```python
from build123d import *

# Parameters (mm, degrees)
BOSS_EXTRUDE1_DEPTH       = 18
SKETCH2_W                 = 22.6
SKETCH2_H                 = 12.7
CUT_EXTRUDE1_DEPTH        = 10
F_4_CLEARANCE_HOLE3_D     = 3.2639
F_4_CLEARANCE_HOLE3_DEPTH = 1.59


with BuildPart() as part:
    # Sketch1 → Boss-Extrude1 (new body)
    with BuildSketch(Plane.XY):
        Polygon((10, -20), (0, -20), (0, 0), (40, 0), (40, -20), (30, -20), (30, -18.41), (38.41, -18.41), (38.41, -1.59), (1.59, -1.59), (1.59, -18.41), (10, -18.41), align=None)
    extrude(amount=BOSS_EXTRUDE1_DEPTH)

    # Sketch2 → Cut-Extrude1 (cut)
    with BuildSketch(Plane(origin=(0, 0, 0), x_dir=(1, 0, 0), z_dir=(0, 1, 0))):
        with Locations((20, -6.35)):
            Rectangle(SKETCH2_W, SKETCH2_H)
    extrude(amount=-CUT_EXTRUDE1_DEPTH, mode=Mode.SUBTRACT)

    # #4 Clearance Hole3
    with Locations(Plane(origin=(0, -18.41, 0), x_dir=(1, 0, 0), z_dir=(0, 1, 0))):
        with Locations((5.795, -9), (34.205, -9)):
            Hole(F_4_CLEARANCE_HOLE3_D / 2, depth=F_4_CLEARANCE_HOLE3_DEPTH)


solid = part.part
```
Geometry: final body of the model. Coordinates: model frame, mm. A direction names the side the tool comes from. Coordinates: 2 decimals unless noted, no trailing zeros. Order: outer loops, then holes, each group sorted by start corner. A loop starts at its lowest first (then second) coordinate and runs counter-clockwise, first axis right, second up. Notation, with made-up numbers: (40, 86) -> (54, 86) arc R20 cw to (54, 99) -> close; hole circle Ø10 at (-38, 58). An arc over 180 degrees is marked (long way). Answer in a Markdown table with one row per item.
Item 1: Access query for faces 1 (the flat face through (4, -18.41, 9)), 2 (the cylindrical face through (7.09, -19.22, 9.99)), 3 (the flat face through (8.7, -1, 6)), 4 (the flat face through (10, -19, 9)), 5 (the flat face through (4, -20, 9)). Directions: +Z, -Z, +X, -X, +Y, -Y. A direction counts if a zero-diameter tool reaches every point of the face in a straight line with its end or side. Return the directions, or none.
Return value:
| item | result |
|---|---|
| face 1 | +Z, -Z |
| face 2 | -Y |
| face 3 | -Z, +Y |
| face 4 | +Z, -Z, -Y |
| face 5 | +Z, -Z, +X, -X, -Y |
Item 2: Contact query for a flat-ended pin moving along its axis: P1, Ø0.8, axis at x = 24.5, y = -1, coming from the -Z side. Output: stop coordinate, or through.
Return value:
| item | result |
|---|---|
| P1 | stops at z = 12.7 |
Item 3: Section D-D on z = 9. Output: boundary loops of the cut face in (x, y), plus the area to 3 significant figures.
Return value:
| item | result |
|---|---|
| outline | (0, -20) -> (4.16, -20) -> (4.16, -18.41) -> (1.59, -18.41) -> (1.59, -1.59) -> (8.7, -1.59) -> (8.7, 0) -> (0, 0) -> close; (7.43, -20) -> (10, -20) -> (10, -18.41) -> (7.43, -18.41) -> close; (30, -20) -> (32.57, -20) -> (32.57, -18.41) -> (30, -18.41) -> close; (31.3, -1.59) -> (38.41, -1.59) -> (38.41, -18.41) -> (35.84, -18.41) -> (35.84, -20) -> (40, -20) -> (40, 0) -> (31.3, 0) -> close |
| area | 103 mm² |
Item 4: Section C-C on y = -9.5. Output: boundary loops of the cut face in (x, z), plus the area to 3 significant figures.
Return value:
| item | result |
|---|---|
| outline | (0, 0) -> (1.59, 0) -> (1.59, 18) -> (0, 18) -> close; (38.41, 0) -> (40, 0) -> (40, 18) -> (38.41, 18) -> close |
| area | 57.2 mm² |
Item 5: Draft query along X for faces 6 (the flat face through (36, -20, 9)), 7 (the flat face through (40, -10, 9)), 8 (the flat face through (31.3, -1, 6)). Return one class per face: released by +X, released by -X, zero draft, split by the parting line, or undercut.
Return value:
| item | result |
|---|---|
| face 6 | zero draft |
| face 7 | released by +X |
| face 8 | undercut |
Item 6: Section B-B on z = 6. Output: boundary loops of the cut face in (x, y).
Return value:
| item | result |
|---|---|
| outline | (0, -20) -> (10, -20) -> (10, -18.41) -> (1.59, -18.41) -> (1.59, -1.59) -> (8.7, -1.59) -> (8.7, 0) -> (0, 0) -> close; (30, -20) -> (40, -20) -> (40, 0) -> (31.3, 0) -> (31.3, -1.59) -> (38.41, -1.59) -> (38.41, -18.41) -> (30, -18.41) -> close |
Item 7: Section A-A on x = 3.5. Output: boundary loops of the cut face in (y, z).
Return value:
| item | result |
|---|---|
| outline | (-20, 0) -> (-18.41, 0) -> (-18.41, 18) -> (-20, 18) -> close; (-1.59, 0) -> (0, 0) -> (0, 18) -> (-1.59, 18) -> close |
Item 8: Ray query, L1, parallel to X at y = -19.25, z = 9; L2, parallel to X at y = -11, z = 12.25; L3, parallel to Y at x = 3, z = 1.25. Return the intervals inside material, ascending.
Return value:
| item | result |
|---|---|
| L1 | x = 0 to 4.16, 7.43 to 10, 30 to 32.57, 35.84 to 40 |
| L2 | x = 0 to 1.59, 38.41 to 40 |
| L3 | y = -20 to -18.41, -1.59 to 0 |
